Geometry: final body of the model. Coordinates: model frame, mm. A direction names the side the tool comes from. Round coordinates to 2 decimals unless told otherwise and drop trailing zeros. Order: outer loops, then holes, each group sorted by start corner. A loop starts at its lowest first (then second) coordinate and runs counter-clockwise, first axis right, second up. Notation, with made-up numbers: (60, 18.25) -> (77, 18.25) arc R10 cw to (77, 33.25) -> close; hole circle Ø10 at (-2, 38.5). An arc over 180 degrees is marked (long way). Put each result on its own line as item: value.
```python
from build123d import *

# Parameters (mm, degrees)
F1_DEPTH = 101.6
F2_W     = 50.8
F2_H     = 25.4
F3_DEPTH = 25.4
F4_W     = 50.8
F4_H     = 25.4
F5_DEPTH = 25.4
F7_DEPTH = 76.2
F8_W     = 50.8
F8_H     = 25.4
F9_DEPTH = 254


with BuildPart() as f1:
    # F0 (on Front) → F1 (new body)
    with BuildSketch(Plane.XZ):
        Polygon((0, 25.4), (0, 0), (25.4, 0), (25.4, -25.4), (50.8, -25.4), (50.8, 0), (120.65, 0), (120.65, -25.4), (146.05, -25.4), (146.05, 0), (171.45, 0), (177.8, 0), (177.8, 25.4), align=None)
    extrude(amount=F1_DEPTH)

    # F2 (on face) → F3 (cut)
    with BuildSketch(Plane.YZ.offset(177.8)):
        with Locations((-50.8, 12.7)):
            Rectangle(F2_W, F2_H)
    extrude(amount=-F3_DEPTH, mode=Mode.SUBTRACT)

    # F4 (on face) → F5 (cut)
    with BuildSketch(Plane(origin=(0, 0, 0), x_dir=(0, -1, 0), z_dir=(-1, 0, 0))):
        with Locations((50.8, 12.7)):
            Rectangle(F4_W, F4_H)
    extrude(amount=-F5_DEPTH, mode=Mode.SUBTRACT)

    # F6 (on face) → F7 (join)
    with BuildSketch(Plane.XY.offset(25.4)):
        Polygon((44.45, 0), (95.25, -101.6), (133.35, 0), align=None)
    extrude(amount=F7_DEPTH)

    # F8 (on Right) → F9 (cut)
    with BuildSketch(Plane.YZ):
        with Locations((-76.2, 63.5)):
            Rectangle(F8_W, F8_H)
    extrude(amount=F9_DEPTH, mode=Mode.SUBTRACT)


solid = f1.part
```
1. Cut plane B-B on y = -68. Return loops of the section in (x, z), and give its area (3 significant figures).
Ans:
outline: (25.4, -25.4) -> (50.8, -25.4) -> (50.8, 0) -> (120.65, 0) -> (120.65, -25.4) -> (146.05, -25.4) -> (146.05, 0) -> (152.4, 0) -> (152.4, 25.4) -> (107.85, 25.4) -> (107.85, 50.8) -> (78.45, 50.8) -> (78.45, 25.4) -> (25.4, 25.4) -> close; (78.45, 76.2) -> (107.85, 76.2) -> (107.85, 101.6) -> (78.45, 101.6) -> close
area: 6,010 mm²
2. Contact query for flat-ended pins moving along their axis: P1, Ø1, axis at x = 51, z = 77, coming from the -Y side; P2, Ø13.5, axis at x = 91, y = -88, coming from the -Z side; P3, Ø6, axis at y = -67, z = 9.5, coming from the +X side; P4, Ø12.5, axis at x = 159.5, z = 18.5, coming from the +Y side. Output: stop coordinate, or through.
Ans:
P1: y = -14.1
P2: z = 0
P3: x = 152.4
P4: y = 0
3. Cut plane D-D on y = -18. Return loops of the section in (x, z).
Ans:
outline: (0, 0) -> (25.4, 0) -> (25.4, -25.4) -> (50.8, -25.4) -> (50.8, 0) -> (120.65, 0) -> (120.65, -25.4) -> (146.05, -25.4) -> (146.05, 0) -> (177.8, 0) -> (177.8, 25.4) -> (126.6, 25.4) -> (126.6, 101.6) -> (53.45, 101.6) -> (53.45, 25.4) -> (0, 25.4) -> close
4. Cut plane A-A on z = -5.5. Return loops of the section in (x, y), and give its area (3 significant figures).
Ans:
outline: (25.4, -101.6) -> (50.8, -101.6) -> (50.8, 0) -> (25.4, 0) -> close; (120.65, -101.6) -> (146.05, -101.6) -> (146.05, 0) -> (120.65, 0) -> close
area: 5,160 mm²
5. Material intervals for probe 1 along X at (y, z) = (-21.5, -15); probe 2 along Z at (x, y) = (150.5, -51.5); probe 3 along X at (y, z) = (-33, 5), sorted ascending.
Ans:
probe 1: 25.4 to 50.8, 120.65 to 146.05
probe 2: 0 to 25.4
probe 3: 25.4 to 152.4
6. Cut plane C-C on x = 21. Return loops of the section in (y, z).
Ans:
outline: (-101.6, 0) -> (-76.2, 0) -> (-76.2, 25.4) -> (-101.6, 25.4) -> close; (-25.4, 0) -> (0, 0) -> (0, 25.4) -> (-25.4, 25.4) -> close
7. Draft query along Z for faces 1 (the face through (92, -65, 50.8)), 2 (the face through (0, -13, 13)), 3 (the face through (38, -61, 25.4)). Return one class per face: +Z half, -Z half, draft (parallel to the pull), parting line (faces both ways), or undercut.
Ans:
face 1: undercut
face 2: draft
face 3: +Z half
8. Set-up query: faces 4 (the face through (13, -76.2, 13)), 5 (the face through (165, -25.4, 13)), 6 (the face through (13, -89, 0)), 7 (the face through (50.8, -50, -13)), 8 (the face through (146.05, -50, -13)). Return all of +Z, -Z, +X, -X, +Y, -Y with unobstructed straight access to the full face (end or side cutting, diameter ignored); none if empty.
Ans:
face 4: +Z, -Z, -X
face 5: +Z, -Z, +X
face 6: -Z, -X, +Y, -Y
face 7: -Z, +Y, -Y
face 8: -Z, +X, +Y, -Y
